```python
from build123d import *

# Parameters (mm, degrees)
F0_W     = 76.2
F0_H     = 76.2
F2_DEPTH = 76.2
F1_W     = 50.8
F1_H     = 25.4
F3_DEPTH = 164.592
F4_W     = 25.4
F4_H     = 25.4
F5_DEPTH = 76.2


with BuildPart() as f2:
    # F0 (on Front) → F2 (new body)
    with BuildSketch(Plane.XZ):
        with Locations((38.1, 38.1)):
            Rectangle(F0_W, F0_H)
    extrude(amount=F2_DEPTH)

    # F1 (on Front) → F3 (cut)
    with BuildSketch(Plane.XZ):
        with Locations((25.4, 12.7)):
            Rectangle(F1_W, F1_H)
    extrude(amount=F3_DEPTH, mode=Mode.SUBTRACT)

    # F4 (on face) → F5 (cut)
    with BuildSketch(Plane.XZ.offset(76.2)):
        with Locations((12.7, 38.1)):
            Rectangle(F4_W, F4_H)
    extrude(amount=-F5_DEPTH, mode=Mode.SUBTRACT)


solid = f2.part
```
The model under review builds one solid part; all positions refer to its coordinate system, in mm. A direction names the side the tool comes from. Coordinates: 2 decimals unless noted, no trailing zeros. Write each loop counter-clockwise with the first axis right and the second up, starting at its lowest first coordinate (ties: lowest second). Pieces come first, ordered by that corner, then holes. Notation, with made-up numbers: (87, 89.25) - (135, 89.25) arc R10 ccw to (135, 93.25) - close; hole circle Ø8 at (33.25, 25). An arc over 180 degrees is marked (long way). Answer in a Markdown table with one row per item. Add a question column.
Q1. Consider section A-A on y = -36.5. Give the boundary of the cut face in (x, z), then the cut area to 3 significant figures.
Q2. Consider section C-C on x = 41.5. Give the boundary of the cut face in (y, z), then the cut area to 3 significant figures.
Q3. Consider section B-B on z = 49. Give the boundary of the cut face in (x, y).
Q4. For faces 1 (the face through (46, -76.2, 47)), 2 (the face through (25.4, -39, 38)), list the 3-axis set-ups (+Z, -Z, +X, -X, +Y, -Y) from which the entire face can be reached by the end or side of a thin tool; tool diameter is ignored.
Q5. Clearance check with flat-ended pins moving along their axes: pin 1 (6 mm diameter, centred on x = 45.5, y = -28.5, fed in from -Z); pin 2 (20.5 mm diameter, centred on y = -21.5, z = 44, fed in from -X); pin 3 (20.5 mm diameter, centred on y = -47, z = 19, fed in from -X); pin 4 (1.5 mm diameter, centred on y = -32.5, z = 12.5, fed in from -X). State where each tip first meets the part, or that it passes through.
Q6. To check wall thickness, follow line 1 along Z through (x, y) = (16, -35); line 2 along Z through (x, y) = (28.5, -14.5). State the ranges of each line that lie inside material, in increasing order. Write a range as from..to.
Answers below:
| question | item | result |
|---|---|---|
| 1 | outline | (0, 50.8) - (25.4, 50.8) - (25.4, 25.4) - (50.8, 25.4) - (50.8, 0) - (76.2, 0) - (76.2, 76.2) - (0, 76.2) - close |
| 1 | area | 3,870 mm² |
| 2 | outline | (-76.2, 25.4) - (0, 25.4) - (0, 76.2) - (-76.2, 76.2) - close |
| 2 | area | 3,870 mm² |
| 3 | outline | (25.4, -76.2) - (76.2, -76.2) - (76.2, 0) - (25.4, 0) - close |
| 4 | face 1 | +Z, -Z, +X, -X, -Y |
| 4 | face 2 | -Z, -X, +Y, -Y |
| 5 | pin 1 | z = 25.4 |
| 5 | pin 2 | x = 0 |
| 5 | pin 3 | x = 25.4 |
| 5 | pin 4 | x = 50.8 |
| 6 | line 1 | 50.8..76.2 |
| 6 | line 2 | 25.4..76.2 |
